Input: part model. Units: mm. Frame: model coordinates. Face numbers are marked on the shaded views. A direction names the side the tool comes from. Give positions to 0.01 mm unless a question says otherwise; leave off trailing zeros. Return JSON: item names as keys, results as strings. Group by question number.
Item 1: Section A-A, the plane z = 0. Count the separate pieces of the cut face and the enclosed holes in it, then the cut area to 3 significant figures.
Item 2: Set-up query: the marked faces 1 and 2. Return all of +Z, -Z, +X, -X, +Y, -Y with unobstructed straight access to the full face (end or side cutting, diameter ignored); none if empty.
Item 3: Pin query (flat end, axial travel): P1, Ø2.5, axis at y = -13, z = 2.5, coming from the -X side; P2, Ø4, axis at y = -1, z = -0.5, coming from the +X side; P3, Ø1.5, axis at x = 2.5, y = 14.5, coming from the -Z side. Return the tip coordinate at first contact, or that it passes through.
Item 4: Mould query, pull axis Z, two halves, no side actions, for the marked faces 3, 4 and 5. Classes: released by +Z, released by -Z, zero draft, split by the parting line, or undercut.
Item 5: Line query: line 1 (Y direction, x = 4.6, z = 0); line 2 (X direction, y = -11, z = 3); line 3 (X direction, y = -9, z = 6). Output: solid intervals per line, ascending. Write a range as [from, to].
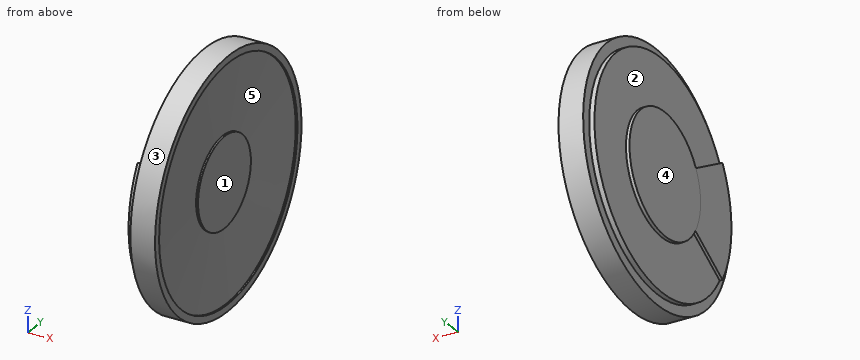
from build123d import *

# Parameters (mm, degrees)
SKETCH2_R           = 8.75
BOSS_EXTRUDE2_DEPTH = 3.5
SKETCH3_R           = 16.5
BOSS_EXTRUDE3_DEPTH = 1.5
SKETCH5_R           = 18
SKETCH5_R_2         = 17
BOSS_EXTRUDE4_DEPTH = 3.55
SKETCH6_R           = 17
SKETCH6_R_2         = 15
BOSS_EXTRUDE5_DEPTH = 1.5
SKETCH8_R           = 6.5
BOSS_EXTRUDE6_DEPTH = 0.75
BOSS_EXTRUDE7_DEPTH = 0.4


with BuildPart() as part:
    # Sketch2 → Boss-Extrude2 (new body)
    with BuildSketch(Plane(origin=(0, 0, 0), x_dir=(0, 0, -1), z_dir=(1, 0, 0))):
        Circle(SKETCH2_R)
    extrude(amount=BOSS_EXTRUDE2_DEPTH)

    # Sketch3 → Boss-Extrude3 (add)
    with BuildSketch(Plane.ZY.offset(-0.5)):
        Circle(SKETCH3_R)
    extrude(amount=-BOSS_EXTRUDE3_DEPTH)



with BuildPart() as body_2:
    # Sketch5 → Boss-Extrude4 (new body)
    with BuildSketch(Plane(origin=(1.25, 0, 0), x_dir=(0, 0, -1), z_dir=(1, 0, 0))):
        Circle(SKETCH5_R)
        Circle(SKETCH5_R_2, mode=Mode.SUBTRACT)
    extrude(amount=BOSS_EXTRUDE4_DEPTH)


with BuildPart() as part_1:
    add(part.part)

    add(body_2.part)  # Boss-Extrude5 merges body 2
    # Sketch6 → Boss-Extrude5 (add)
    with BuildSketch(Plane(origin=(1.25, 0, 0), x_dir=(0, 0, -1), z_dir=(1, 0, 0))):
        Circle(SKETCH6_R)
        Circle(SKETCH6_R_2, mode=Mode.SUBTRACT)
    extrude(amount=BOSS_EXTRUDE5_DEPTH)

    # Sketch8 → Boss-Extrude6 (add)
    with BuildSketch(Plane(origin=(3.5, 0, 0), x_dir=(0, 0, -1), z_dir=(1, 0, 0))):
        Circle(SKETCH8_R)
    extrude(amount=BOSS_EXTRUDE6_DEPTH)

    # Sketch10 → Revolve1 (revolve)
    with BuildSketch(Plane(origin=(0, 0, 0), x_dir=(1, 0, 0), z_dir=(0, 1, 0))):
        Polygon((1.25, 0), (3.611187211, 0), (4.55, 17), (2.75, 17), align=None)
    revolve(axis=Axis((1.25, 0, 0), (1, 0, 0)))

    # Sketch11 → Boss-Extrude7 (add)
    with BuildSketch(Plane.ZY.offset(-0.5)):
        with BuildLine():
            Line((8.25, -14.289419162), (4.375, -7.577722283))
            ThreePointArc((4.375, -7.577722283), (0, -8.75), (-4.375, -7.577722283))
            Line((-4.375, -7.577722283), (-8.25, -14.289419162))
            ThreePointArc((-8.25, -14.289419162), (0, -16.5), (8.25, -14.289419162))
        make_face()
    extrude(amount=BOSS_EXTRUDE7_DEPTH)


solid = part_1.part
Answer below:
{
 "1": {"separate pieces": "1", "enclosed holes": "2", "area": "142 mm2"},
 "2": {"face 1": "+X", "face 2": "-X"},
 "3": {"P1": "stops at x = 0.1", "P2": "stops at x = 4.25", "P3": "stops at z = -11.62"},
 "4": {"face 3": "split by the parting line", "face 4": "zero draft", "face 5": "undercut"},
 "5": {"line 1": "y = [-18, -17], [17, 18]", "line 2": "x = [0.1, 2], [2.26, 4.24]", "line 3": "x = [0.5, 2], [2.2, 4.21]"}
}
